For this review, take the finished solid that the model builds, in its own axes (mm). Face numbers are marked on the shaded views. A direction names the side the tool comes from. Give positions to 0.01 mm unless a question says otherwise; leave off trailing zeros. Write each loop counter-clockwise with the first axis right and the second up, starting at its lowest first coordinate (ties: lowest second). Pieces come first, ordered by that corner, then holes. Notation, with made-up numbers: M 7,-13.75 L 62,-13.75 A24 ccw 62,-1.75 Z; hole C 37.25,25.25 d9. An arc over 180 degrees is marked long. Use one line per item in the form item = value. Start each with the question number.
Q1. Consider section D-D on x = 0. Write out the cut boundary in (y, z).
Q2. Clearance check with flat-ended pins moving along their axes: pin 1 Ø5 at (x, z) = (68.5, 110.5) entering from -Y; pin 2 Ø10 at (x, z) = (15, -72.5) entering from +Y; pin 3 Ø15 at (x, z) = (79.5, 16) entering from +Y. State where each tip first meets the part, or that it passes through.
Q3. Consider section A-A on x = 70. Write out the cut boundary in (y, z).
Q4. For probe 1 along Z at (x, y) = (85, 79.5); probe 2 along Y at (x, z) = (0, -109.5); probe 3 along X at (y, z) = (25.4, -111), list the stretches that pass through material, from the lowest coordinate up. Write a range as [from, to].
Q5. Consider section C-C on x = -25. Write out the cut boundary in (y, z).
Q6. Mouldability with a two-part tool opening along Y and no side actions: class the marked faces 3, 4 and 5 as released by +Y, released by -Y, zero draft, split by the parting line, or undercut.
Q7. Tool access review of the marked faces 1 and 2: name each direction out of +Z, -Z, +X, -X, +Y, -Y from which nothing blocks a thin tool from reaching the whole face with its end or side.
Q8. Consider section B-B on z = -66.5. Write out the cut boundary in (x, y), and give its area (3 significant figures).
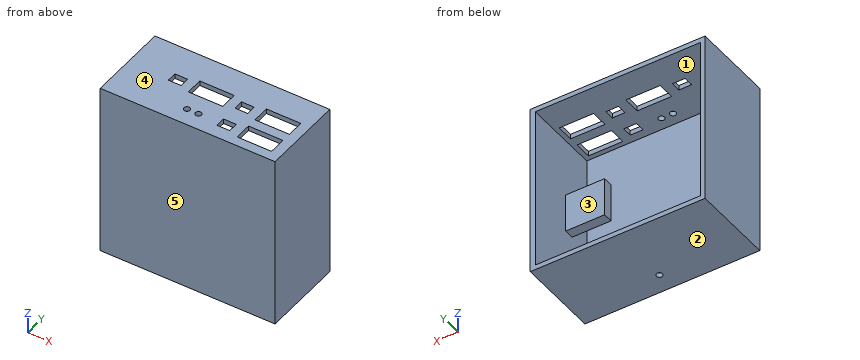
Autodesk Inventor part; units mm, degrees
ref_plane "YZ Plane" through (0, 0, 0) normal (1, 0, 0) x (0, 1, 0)
ref_plane "XZ Plane" through (0, 0, 0) normal (0, 1, 0) x (-1, 0, 0)
ref_plane "XY Plane" through (0, 0, 0) normal (0, 0, 1) x (1, 0, 0)
sketch "Sketch1" plane through (0, 0, 0) normal (0, 1, 0) x (-1, 0, 0)
  line L0 (0, 0) -> (-114.3, 0)
  line L1 (-114.3, 0) -> (-114.3, -114.3)
  line L2 (-114.3, -114.3) -> (114.3, -114.3)
  line L3 (114.3, -114.3) -> (114.3, 114.3)
  line L4 (114.3, 114.3) -> (-114.3, 114.3)
  line L5 (-114.3, 114.3) -> (-114.3, 0)
  dimension "d0" = 114.3
  dimension "d1" = 114.3
  dimension "d2" = 228.6
  dimension "d3" = 228.6
  dimension "d4" = 90
extrude "Extrusion1" add sketch "Sketch1" along normal blind 6.35
sketch "Sketch3" plane through (0, 6.35, 0) normal (0, 1, 0) x (1, 0, 0)
  line L0 (114.3, 114.3) -> (-114.3, 114.3)
  line L1 (-114.3, 114.3) -> (-108.2442, 114.3)
  line L2 (-108.2442, 114.3) -> (-108.2442, -114.3)
  line L3 (-108.2442, 114.3) -> (120.3558, 114.3) construction
  line L4 (-108.2442, -114.3) -> (-108.2442, -107.95)
  line L5 (-108.2442, -107.95) -> (107.6558, -107.95)
  line L6 (107.6558, -107.95) -> (107.6558, 107.95)
  line L7 (107.6558, 107.95) -> (-108.2442, 107.95)
  line L8 (-114.3, 114.3) -> (-114.3, -114.3)
  line L9 (-114.3, -114.3) -> (114.3, -114.3)
  line L10 (114.3, -114.3) -> (114.3, 114.3)
  point P0 (0, 0)
  dimension "d19" = 228.6
  dimension "d20" = 90
  dimension "d21" = 6.35
  dimension "d22" = 215.9
  dimension "d23" = 215.9
extrude "Extrusion3" add sketch "Sketch3" along normal blind 101.6 contours L10 L9 L2 L5 L6 L7 L0 | L2 L9 L8 L0
sketch "Sketch4" plane through (-114.3, 0, 114.3) normal (0, 0, 1) x (1, 0, 0)
  line L0 (221.9558, 6.35) -> (221.9558, 107.95)
  line L1 (221.9558, 107.95) -> (221.9558, 44.45)
  line L2 (221.9558, 6.35) -> (6.0558, 6.35)
  line L3 (221.9558, 6.35) -> (221.9558, 12.7)
  line L4 (221.9558, 6.35) -> (221.9558, 107.95)
  line L5 (221.9558, 12.7) -> (215.6058, 12.7)
  line L6 (215.6058, 12.7) -> (215.6058, 35.2044)
  line L7 (215.6058, 35.2044) -> (170.597, 35.2044)
  line L8 (170.597, 35.2044) -> (170.597, 12.7)
  line L9 (170.597, 12.7) -> (215.6058, 12.7)
  line L10 (170.597, 12.7) -> (157.897, 12.7)
  line L11 (157.897, 12.7) -> (157.897, 35.2044)
  line L12 (157.897, 35.2044) -> (112.8882, 35.2044)
  line L13 (112.8882, 35.2044) -> (112.8882, 12.7)
  line L14 (112.8882, 12.7) -> (157.897, 12.7)
  line L15 (112.8882, 35.2044) -> (100.1882, 35.2044)
  line L16 (100.1882, 35.2044) -> (100.1882, 12.7)
  line L17 (100.1882, 12.7) -> (55.1794, 12.7)
  line L18 (55.1794, 12.7) -> (55.1794, 35.2044)
  line L19 (55.1794, 35.2044) -> (100.1882, 35.2044)
  line L20 (215.6058, 35.2044) -> (215.6058, 47.9044)
  line L21 (215.6058, 47.9044) -> (170.597, 47.9044)
  line L22 (170.597, 47.9044) -> (170.597, 70.4088)
  line L23 (170.597, 70.4088) -> (215.6058, 70.4088)
  line L24 (215.6058, 70.4088) -> (215.6058, 47.9044)
  line L25 (215.6058, 70.4088) -> (215.6058, 83.1088)
  point P0 (114.3, 0)
  point P1 (215.6058, 105.6132)
  point P2 (170.597, 105.6132)
  point P3 (170.597, 83.1088)
  dimension "d34" = 6.35
  dimension "d35" = 6.35
  dimension "d36" = 22.5044
  dimension "d37" = 45.0088
  dimension "d38" = 12.7
  dimension "d39" = 45.0088
  dimension "d40" = 12.7
  dimension "d41" = 45.0088
  dimension "d44" = 12.7
  dimension "d45" = 22.5044
  dimension "d46" = 12.7
  dimension "d47" = 22.5044
sketch "Sketch9" plane through (-114.3, 0, 114.3) normal (0, 0, 1) x (1, 0, 0)
  line L0 (170.597, 47.9044) -> (170.597, 70.4088)
  line L1 (170.597, 70.4088) -> (170.597, 59.1566)
  line L2 (170.597, 59.1566) -> (157.897, 59.1566)
  line L3 (170.597, 35.0034) -> (170.597, 23.7512)
  line L4 (170.597, 23.7512) -> (157.897, 23.7512)
  line L5 (157.897, 59.1566) -> (157.897, 65.6066)
  line L6 (157.897, 65.6066) -> (141.197, 65.6066)
  line L7 (141.197, 65.6066) -> (141.197, 52.7034)
  line L8 (141.197, 52.7034) -> (157.897, 52.7034)
  line L9 (157.897, 52.7034) -> (157.897, 59.1566)
  line L10 (157.897, 23.7512) -> (157.897, 30.2012)
  line L11 (157.897, 30.2012) -> (141.197, 30.2012)
  line L12 (141.197, 30.2012) -> (141.197, 17.3012)
  line L13 (141.197, 17.3012) -> (157.897, 17.3012)
  line L14 (157.897, 17.3012) -> (157.897, 23.7512)
  point P0 (114.3, 0)
  point P1 (170.597, 105.6132)
  dimension "d64" = 11.2522
  dimension "d65" = 12.7
  dimension "d67" = 11.2522
  dimension "d68" = 12.7
  dimension "d82" = 6.45
  dimension "d83" = 12.9032
  dimension "d84" = 6.45
  dimension "d85" = 12.9
extrude "Extrusion4" cut sketch "Sketch4" against normal blind 114.3 contours L9 L8 L7 L6 | L21 L22 L23 L24
extrude "Extrusion6" cut sketch "Sketch9" against normal blind 114.3
sketch "Sketch14" plane through (-108.2442, 6.35, 107.95) normal (1, 0, 0) x (0, 0, -1)
  line L0 (215.9, 0) -> (0, 0)
  line L1 (0, 0) -> (0, 101.6)
  line L2 (-6.35, 101.6) -> (0, 101.6)
  line L3 (0, 101.6) -> (215.9, 101.6)
  line L4 (215.9, 0) -> (215.9, 101.6)
  line L5 (215.9, 66.675) -> (215.9, 9.525)
  line L6 (215.9, 66.675) -> (203.2, 66.675)
  line L7 (203.2, 66.675) -> (203.2, 9.525)
  line L8 (203.2, 9.525) -> (158.75, 9.525)
  line L9 (158.75, 9.525) -> (158.75, 66.675)
  line L10 (158.75, 66.675) -> (203.2, 66.675)
  line L11 (158.75, 66.675) -> (146.05, 66.675)
  line L12 (146.05, 66.675) -> (146.05, 9.525)
  line L13 (146.05, 9.525) -> (101.6, 9.525)
  line L14 (101.6, 9.525) -> (101.6, 66.675)
  line L15 (101.6, 66.675) -> (146.05, 66.675)
  line L16 (101.6, 66.675) -> (88.9, 66.675)
  line L17 (88.9, 66.675) -> (88.9, 9.525)
  line L18 (88.9, 9.525) -> (44.45, 9.525)
  line L19 (44.45, 9.525) -> (44.45, 66.675)
  line L20 (44.45, 66.675) -> (88.9, 66.675)
  line L21 (203.2, 66.675) -> (180.975, 66.675)
  line L22 (180.975, 66.675) -> (180.975, 61.675)
  line L23 (180.975, 9.525) -> (180.975, 14.525)
  circle A0 centre (180.975, 61.675) radius 2.54
  circle A1 centre (180.975, 14.525) radius 2.54
  line L24 (123.825, 66.675) -> (123.825, 61.675)
  line L25 (123.825, 9.525) -> (123.825, 14.525)
  circle A2 centre (123.825, 61.675) radius 2.54
  circle A3 centre (123.825, 14.525) radius 2.54
  line L26 (66.675, 66.675) -> (66.675, 61.675)
  line L27 (66.675, 9.525) -> (66.675, 14.525)
  circle A4 centre (66.675, 61.675) radius 2.54
  circle A5 centre (66.675, 14.525) radius 2.54
  point P0 (107.95, -6.35)
  dimension "d123" = 57.15
  dimension "d124" = 12.7
  dimension "d125" = 44.45
  dimension "d126" = 12.7
  dimension "d127" = 44.45
  dimension "d128" = 12.7
  dimension "d129" = 44.45
  dimension "d139" = 22.225
  dimension "d140" = 5
  dimension "d141" = 5
  dimension "d142" = 5.08
  dimension "d143" = 5.08
  dimension "d144" = 5
  dimension "d145" = 5
  dimension "d146" = 5.08
  dimension "d147" = 5.08
  dimension "d148" = 5
  dimension "d149" = 5
  dimension "d150" = 5.08
  dimension "d151" = 5.08
sketch "Sketch15" plane through (-114.3, 0, 114.3) normal (0, 0, 1) x (1, 0, 0)
  line L0 (141.197, 65.6066) -> (141.197, 52.7034)
  line L1 (141.197, 59.155) -> (128.497, 59.155)
  line L2 (128.497, 59.155) -> (128.497, 70.4088)
  line L3 (128.497, 70.4088) -> (128.497, 47.9044)
  line L4 (215.6058, 47.9044) -> (170.597, 47.9044)
  line L5 (128.497, 47.9044) -> (83.4882, 47.9044)
  line L6 (83.4882, 47.9044) -> (83.4882, 70.4088)
  line L7 (83.4882, 70.4088) -> (128.497, 70.4088)
  line L8 (83.4882, 59.1566) -> (70.7882, 59.1566)
  line L9 (70.7882, 59.1566) -> (70.7882, 65.6066)
  line L10 (70.7882, 65.6066) -> (70.7882, 52.7034)
  line L11 (70.7882, 52.7034) -> (70.7882, 59.1566)
  line L12 (70.7882, 52.7034) -> (54.1004, 52.7034)
  line L13 (54.1004, 52.7034) -> (54.1004, 65.6066)
  line L14 (54.1004, 65.6066) -> (70.7882, 65.6066)
  point P0 (114.3, 0)
  dimension "d115" = 12.7
  dimension "d116" = 45.0088
  dimension "d117" = 12.7
  dimension "d118" = 16.6878
extrude "Extrusion9" cut sketch "Sketch15" against normal blind 114.3
sketch "Sketch16" plane through (-114.3, 0, 114.3) normal (0, 0, 1) x (1, 0, 0)
  line L0 (83.4882, 70.4088) -> (83.4882, 47.9044)
  line L1 (83.4882, 47.9044) -> (98.4911, 47.9044)
  line L2 (98.4911, 47.9044) -> (113.4941, 47.9044)
  line L3 (128.497, 47.9044) -> (83.4882, 47.9044)
  line L4 (113.4941, 47.9044) -> (128.497, 47.9044)
  line L5 (98.4911, 47.9044) -> (98.4911, 22.5044)
  line L6 (113.4941, 47.9044) -> (113.4941, 22.5044)
  circle A0 centre (98.4911, 22.5044) radius 4
  circle A1 centre (113.4941, 22.5044) radius 4
  point P0 (114.3, 0)
  dimension "d130" = 15.0029
  dimension "d131" = 15.0029
  dimension "d132" = 15.0029
  dimension "d133" = 25.4
  dimension "d134" = 25.4
  dimension "d135" = 8
  dimension "d136" = 8
extrude "Extrusion10" cut sketch "Sketch16" against normal blind 76.2
sketch "Sketch17" plane through (0, 6.35, 0) normal (0, 1, 0) x (1, 0, 0)
  line L0 (107.6558, -107.95) -> (94.9558, -107.95)
  line L1 (107.6558, 107.95) -> (107.6558, -107.95)
  line L2 (107.6558, -107.95) -> (120.3558, -107.95) construction
  line L3 (94.9558, -6.35) -> (94.9558, 19.05)
  line L4 (94.9558, 19.05) -> (94.9558, 44.45)
  line L5 (94.9558, 44.45) -> (94.9558, 69.85)
  line L6 (94.9558, 69.85) -> (94.9558, 95.25)
  circle A0 centre (94.9558, -6.35) radius 2.54
  circle A1 centre (94.9558, 19.05) radius 2.54
  circle A2 centre (94.9558, 44.45) radius 2.54
  circle A3 centre (94.9558, 69.85) radius 2.54
  line L7 (-108.2442, -107.95) -> (-82.8442, -107.95)
  line L8 (107.6558, -107.95) -> (-108.2442, -107.95)
  line L9 (-82.8442, -107.95) -> (-82.8442, -95.25)
  line L10 (-82.8442, -95.25) -> (-82.8442, -82.55)
  line L11 (-82.8442, -82.55) -> (-82.8442, -69.85)
  circle A4 centre (-82.8442, -95.25) radius 2.54
  circle A5 centre (-82.8442, -82.55) radius 2.54
  circle A6 centre (-82.8442, -69.85) radius 2.54
  point P0 (0, 0)
  dimension "d152" = 12.7
  dimension "d153" = 180
  dimension "d159" = 25.4
  dimension "d161" = 25.4
  dimension "d162" = 25.4
  dimension "d163" = 25.4
  dimension "d164" = 5.08
  dimension "d165" = 5.08
  dimension "d166" = 5.08
  dimension "d167" = 5.08
  dimension "d173" = 25.4
  dimension "d174" = 12.7
  dimension "d175" = 12.7
  dimension "d176" = 12.7
  dimension "d177" = 5.08
  dimension "d178" = 5.08
  dimension "d179" = 5.08
sketch "Sketch18" plane through (0, 6.35, 0) normal (0, 1, 0) x (1, 0, 0)
  line L0 (-8.3074, -72.1776) -> (-8.3074, -114.3)
  line L1 (14.197, -114.3) -> (-30.8118, -114.3)
  line L2 (-8.3074, -114.3) -> (-8.3074, 38.1)
  line L3 (-8.3074, 38.1) -> (-33.7074, 38.1)
  line L4 (-33.7074, 38.1) -> (17.0926, 38.1)
  circle A0 centre (-33.7074, 38.1) radius 2.54
  circle A1 centre (-8.3074, 38.1) radius 2.54
  circle A2 centre (17.0926, 38.1) radius 2.54
  point P0 (0, 0)
  dimension "d180" = 152.4
  dimension "d181" = 25.4
  dimension "d182" = 50.8
  dimension "d183" = 5.08
  dimension "d184" = 5.08
  dimension "d185" = 5.08
sketch "Sketch19" plane through (107.6558, 6.35, -107.95) normal (-1, 0, 0) x (0, 0, 1)
  line L0 (215.9, 41.5544) -> (88.9, 41.5544)
  line L1 (88.9, 41.5544) -> (139.7, 41.5544)
  line L2 (215.9, 28.8544) -> (88.9, 28.8544)
  line L3 (88.9, 28.8544) -> (139.7, 28.8544)
  line L4 (139.7, 41.5544) -> (139.7, 28.8544)
  line L5 (88.9, 41.5544) -> (88.9, 28.8544)
  point P0 (107.95, -6.35)
  dimension "d186" = 127
  dimension "d187" = 50.8
  dimension "d188" = 127
extrude "Extrusion11" add sketch "Sketch19" along normal blind 50.8
sketch "Sketch21" plane through (114.3, 0, -114.3) normal (0, 0, -1) x (-1, 0, 0)
  line L0 (114.3, 0) -> (114.3, 25.4)
  arc A0 (114.3, 25.4) -> (46.4215, 144.8435) centre (-24.7297, 25.4) ccw
  circle A1 centre (114.3, 25.4) radius 2.54
  circle A2 centre (114.3, 25.4) radius 4
  dimension "d195" = 25.4
  dimension "d196" = 5.08
  dimension "d197" = 8
extrude "Extrusion13" cut sketch "Sketch21" against normal blind 50.8
properties part number "box thin walled"
Working result:
q1.outline = M 0,-114.3 L 21.4,-114.3 L 21.4,-107.95 L 6.35,-107.95 L 6.35,107.95 L 18.59,107.95 L 18.59,114.3 L 0,114.3 Z; M 26.42,107.95 L 47.9,107.95 L 47.9,114.3 L 26.42,114.3 Z; M 29.4,-114.3 L 107.95,-114.3 L 107.95,-107.95 L 29.4,-107.95 Z; M 70.41,107.95 L 107.95,107.95 L 107.95,114.3 L 70.41,114.3 Z
q2.pin_1 = 0
q2.pin_2 = 6.35
q2.pin_3 = 47.9
q3.outline = M 0,-114.3 L 107.95,-114.3 L 107.95,-107.95 L 6.35,-107.95 L 6.35,107.95 L 12.7,107.95 L 12.7,114.3 L 0,114.3 Z; M 35.2,-19.05 L 47.9,-19.05 L 47.9,31.75 L 35.2,31.75 Z; M 35.2,107.95 L 47.9,107.95 L 47.9,114.3 L 35.2,114.3 Z; M 70.41,107.95 L 107.95,107.95 L 107.95,114.3 L 70.41,114.3 Z
q4.probe_1 = [-114.3, -107.95], [107.95, 114.3]
q4.probe_2 = [0, 21.4], [29.4, 107.95]
q4.probe_3 = [-114.3, -4], [4, 114.3]
q5.outline = M 0,-114.3 L 107.95,-114.3 L 107.95,-107.95 L 6.35,-107.95 L 6.35,107.95 L 47.9,107.95 L 47.9,114.3 L 0,114.3 Z; M 70.41,107.95 L 107.95,107.95 L 107.95,114.3 L 70.41,114.3 Z
q6.face_3 = released by +Y
q6.face_4 = zero draft
q6.face_5 = released by -Y
q7.face_1 = +Y
q7.face_2 = -Z, +X, -X, +Y, -Y
q8.outline = M -114.3,0 L 114.3,0 L 114.3,107.95 L 107.66,107.95 L 107.66,6.35 L -108.24,6.35 L -108.24,107.95 L -114.3,107.95 Z
q8.area = 2,740 mm²
